from build123d import *

# Parameters (mm, degrees)
EXTRUDE_TOOTH_DEPTH = 3
PATTERN_TEETH_COUNT = 20
PATTERN_TEETH_PITCH = 4


with BuildPart() as part:
    # Sketch1 → Extrude Tooth (new, symmetric)
    with BuildSketch(Plane.XY):
        Polygon((-0.483692342, 2.2), (0.483692342, 2.2), (1.50956919, 0), (2, 0), (2, -3), (-2, -3), (-2, 0), (-1.50956919, 0), align=None)
    extrude_tooth = extrude(amount=EXTRUDE_TOOTH_DEPTH, both=True)

    # Pattern Teeth: Extrude Tooth ×20
    with Locations(*[(i * PATTERN_TEETH_PITCH, 0, 0) for i in range(1, PATTERN_TEETH_COUNT)]):
        add(extrude_tooth)


solid = part.part
Work out the finished part from the listing and answer in its coordinate system (mm). Coordinates: 2 decimals unless noted, no trailing zeros.
1. For a pull along X with two mould halves and no side action, classify faces 1 (the flat face through (39, -3, 0)), 2 (the flat face through (12.989, 1.115, 0.042)), 3 (the flat face through (14.996, 1.085, 0.042)) as +X half, -X half, draft (parallel to the pull), parting line (faces both ways), or undercut.
Results list:
face 1: draft
face 2: undercut
face 3: undercut
2. Flat-ended cylindrical pins translate along their axes: pin 1 (1.1 mm diameter, centred on x = 46, z = 0.5, fed in from +Y); pin 2 (0.5 mm diameter, centred on x = 66, z = -1, fed in from +Y); pin 3 (2 mm diameter, centred on x = 31, z = -1.5, fed in from +Y). Find the tip coordinate at first contact, or state that the pin passes through.
Results list:
pin 1: stops at y = 0.13
pin 2: stops at y = 0
pin 3: stops at y = 2.2
3. Consider line 1 along Y through (x, z) = (26, 0.85); line 2 along Y through (x, z) = (20.5, 0.5). Determine where each line is inside the solid, lowest interval first.
Results list:
line 1: y = -3 to 0
line 2: y = -3 to 2.17
4. The part is cut by section A-A, the plane y = 1.35. State how many separate pieces and enclosed holes the cut face has, and give its area (3 significant figures).
Results list:
separate pieces: 20
enclosed holes: 0
area: 211 mm2
